Model file for the job. Use its own axes, mm. A direction names the side the tool comes from. Coordinates: 2 decimals unless noted, no trailing zeros. Order: outer loops, then holes, each group sorted by start corner. A loop starts at its lowest first (then second) coordinate and runs counter-clockwise, first axis right, second up. Notation, with made-up numbers: (61.25, 17.5) -> (115.25, 17.5) arc R31 cw to (115.25, 54.5) -> close; hole circle Ø9 at (44.25, -28.75). An arc over 180 degrees is marked (long way). Write item = value, one per line. Start each with the question number.
Q1. Cut at D-D, the plane x = -43.5. List the corners of the cut face in (y, z), plus the area to 3 significant figures.
Q2. Flat gauge pins, fed straight in: pin 1 (13 mm diameter, centred on y = 15, z = -75, fed in from -X); pin 2 (1.5 mm diameter, centred on x = -11.5, y = 8, fed in from +Z). Where does each tip first touch, or does it go through?
Q3. Cut at C-C, the plane z = 42. List the corners of the cut face in (x, y).
Q4. Wall check: line 1 (Z direction, x = -68.55, y = 15); line 2 (X direction, y = 19.75, z = 30); line 3 (Z direction, x = -47.5, y = 24). Give the ranges that are in metal, low to high. Write a range as from..to.
Q5. 3-axis set-ups, long thin cutter, end or side, ignore diameter. For faces 1 (the face through (-1, 17, -93)), 2 (the face through (-1, 17, -95)), 3 (the face through (1, 2, 1)): which of +Z, -Z, +X, -X, +Y, -Y reach the whole face in a straight line?
Q6. Mould opens along Y. For faces 4 (the face through (1, 5, -90)), 5 (the face through (0.95, 6.35, -88.52)), 6 (the face through (-1, 27, -93)), 7 (the face through (-0.95, 6.35, 88.52)) say: +Y half, -Y half, draft (parallel to the pull), parting line (faces both ways), or undercut.
Q7. Cut at B-B, the plane y = 22.25. List the corners of the cut face in (x, z), plus the area to 3 significant figures.
Q8. Cut at A-A, the plane z = -75. List the corners of the cut face in (x, y), plus the area to 3 significant figures.
Autodesk Inventor part; units mm, degrees
ref_plane "YZ Plane" through (0, 0, 0) normal (1, 0, 0) x (0, 1, 0)
ref_plane "XZ Plane" through (0, 0, 0) normal (0, 1, 0) x (-1, 0, 0)
ref_plane "XY Plane" through (0, 0, 0) normal (0, 0, 1) x (1, 0, 0)
sketch "Esquisse1" plane through (0, 0, 0) normal (0, 1, 0) x (-1, 0, 0)
  line L0 (-70, 95) -> (70, 95)
  line L1 (70, 95) -> (70, -95)
  line L2 (70, -95) -> (-70, -95)
  line L3 (-70, -95) -> (-70, 95)
  line L4 (-70, 95) -> (70, -95) construction
  line L5 (70, 95) -> (-70, -95) construction
  point P0 (0, 0)
  dimension "d0" = 140
  dimension "d1" = 190
extrude "Extrusion1" add sketch "Esquisse1" along normal blind 30
chamfer "Chanfrein1" distance 10 angle 45 2 edges at (0, 0, 95) (0, 0, -95)
chamfer "Chanfrein2" distance 5 angle 45 2 edges at (0, 30, 95) (0, 30, -95)
shell "Coque1" thickness 2 removed faces 1 at (23.3333, 30, 30)
sketch "Esquisse2" plane through (70, 0, 85) normal (1, 0, 0) x (0, 0, -1)
  line L0 (-10, 10) -> (-10, 25)
  line L1 (180, 10) -> (180, 25)
  line L2 (-5, 30) -> (175, 30)
  line L3 (170, 0) -> (0, 0)
  circle A0 centre (10, 15) radius 5
  line L4 (85, 0) -> (85, 30)
  circle A1 centre (160, 15) radius 5
  dimension "d11" = 10
  dimension "d12" = 20
  dimension "d13" = 15
extrude "Extrusion2" cut sketch "Esquisse2" against normal blind 3
ref_plane "Plan de construction1" through (0, 0, 85) normal (1, 0, 0) x (0, 0, -1)
mirror "Symétrie1" about plane through (0, 0, 85) normal (1, 0, 0) of "Extrusion2"
properties part number "Chassis"
Here are the results:
q1.outline = (0, -85) -> (10, -95) -> (25, -95) -> (30, -90) -> (30, -87.17) -> (24.17, -93) -> (10.83, -93) -> (2, -84.17) -> (2, 84.17) -> (10.83, 93) -> (24.17, 93) -> (30, 87.17) -> (30, 90) -> (25, 95) -> (10, 95) -> (0, 85) -> close
q1.area = 479 mm²
q2.pin_1 = -70
q2.pin_2 = 93.75
q3.outline = (-70, 0) -> (70, 0) -> (70, 30) -> (68, 30) -> (68, 2) -> (-68, 2) -> (-68, 30) -> (-70, 30) -> close
q4.line_1 = -95..-80, -70..70, 80..95
q4.line_2 = -70..-68, 68..70
q4.line_3 = -95..-93, 93..95
q5.face_1 = none
q5.face_2 = -Z, +X, -X, +Y, -Y
q5.face_3 = +Y
q6.face_4 = -Y half
q6.face_5 = undercut
q6.face_6 = +Y half
q6.face_7 = undercut
q7.outline = (-70, -95) -> (70, -95) -> (70, 95) -> (-70, 95) -> close; hole (-68, -93) -> (68, -93) -> (68, 93) -> (-68, 93) -> close
q7.area = 1,300 mm²
q8.outline = (-70, 0) -> (70, 0) -> (70, 10) -> (68, 10) -> (68, 2) -> (-68, 2) -> (-68, 10) -> (-70, 10) -> close; (-70, 20) -> (-68, 20) -> (-68, 30) -> (-70, 30) -> close; (68, 20) -> (70, 20) -> (70, 30) -> (68, 30) -> close
q8.area = 352 mm²
